For this review, take the finished solid that the model builds, in its own axes (mm). Face numbers are marked on the shaded views. Round coordinates to 2 decimals unless told otherwise and drop trailing zeros. Write each loop counter-clockwise with the first axis right and the second up, starting at its lowest first coordinate (ties: lowest second). Pieces come first, ordered by that corner, then holes. Notation, with made-up numbers: (32.5, -19.5) -> (77.5, -19.5) arc R24 cw to (77.5, 5.5) -> close; hole circle Ø5 at (23, 40). An arc over 180 degrees is marked (long way). Answer as CSV lines item,"result". Start each with the question number.
Item 1: For pin 1 Ø1.1 at (x, y) = (32, 1) entering from -Z; pin 2 Ø3 at (x, z) = (8, 8.5) entering from -Y; pin 3 Ø4 at (x, z) = (35, 3) entering from +Y, all flat-tipped, find the tip position at first contact; note any pin that passes through.
Item 2: Take a section at C-C on x = 37.5. Give the boundary of the cut face in (y, z), then the cut area to 3 significant figures.
Item 3: Take a section at A-A on x = 9. Give the boundary of the cut face in (y, z).
Item 4: Take a section at B-B on y = 0.6. Give the boundary of the cut face in (x, z), then the cut area to 3 significant figures.
Item 5: Take a section at D-D on z = 16.25. Give the boundary of the cut face in (x, y), then the cut area to 3 significant figures.
Item 6: Wall thickness on probe 1 along X at (y, z) = (1.15, 9); probe 2 along Y at (x, z) = (15, 12.75); probe 3 along X at (y, z) = (1.7, 13): over which ranges is each line inside the solid? List them lowest first. Write a range as from..to.
Item 7: Mouldability with a two-part tool opening along X and no side actions: class the marked faces 1 and 2 as +X half, -X half, draft (parallel to the pull), parting line (faces both ways), or undercut.
```python
from build123d import *

# Parameters (mm, degrees)
F0_W     = 42
F0_H     = 18
F2_DEPTH = 1.91
F1_R     = 4.6
F3_DEPTH = 3.18
F4_SIZE  = 0.25


# Not quite as in the source:
# - a feature names something its author has since deleted; it is built from what else it names


with BuildPart() as f2:
    # F0 (on Front) → F2 (new body)
    with BuildSketch(Plane.XZ):
        with Locations((21, 9)):
            Rectangle(F0_W, F0_H)
        with BuildLine():
            ThreePointArc((11.1703455946, 12.36), (9, 5), (6.8296544054, 12.36))
            ThreePointArc((6.8296544054, 12.36), (7.0893980916, 12.4791663047), (7.372240804, 12.52))
            Line((7.372240804, 12.52), (10.627759196, 12.52))
            ThreePointArc((10.627759196, 12.52), (10.9106019084, 12.4791663047), (11.1703455946, 12.36))
        make_face(mode=Mode.SUBTRACT)
        with BuildLine():
            Line((32.5, 3.2), (31.5, 3.2))
            ThreePointArc((31.5, 3.2), (27.3987806691, 4.8987806691), (25.7, 9))
            ThreePointArc((25.7, 9), (27.3987806691, 13.1012193309), (31.5, 14.8))
            Line((31.5, 14.8), (32.5, 14.8))
            ThreePointArc((32.5, 14.8), (36.6012193309, 13.1012193309), (38.3, 9))
            ThreePointArc((38.3, 9), (36.6012193309, 4.8987806691), (32.5, 3.2))
        make_face(mode=Mode.SUBTRACT)
    extrude(amount=-F2_DEPTH)

    # F1 (on face) → F3 (join)
    with BuildSketch(Plane.XZ):
        with Locations((9, 9)):
            Circle(F1_R)
        with BuildLine():
            ThreePointArc((10.627759196, 12.52), (10.9106019084, 12.4791663047), (11.1703455946, 12.36))
            ThreePointArc((11.1703455946, 12.36), (9, 5), (6.8296544054, 12.36))
            ThreePointArc((6.8296544054, 12.36), (7.0893980916, 12.4791663047), (7.372240804, 12.52))
            Line((7.372240804, 12.52), (10.627759196, 12.52))
        make_face(mode=Mode.SUBTRACT)
    extrude(amount=-F3_DEPTH)

    # F4
    f4_edges = [f2.edges().sort_by_distance(p)[0] for p in [
        (4.4, 3.18, 9),
    ]]
    chamfer(f4_edges, length=F4_SIZE)


solid = f2.part
```
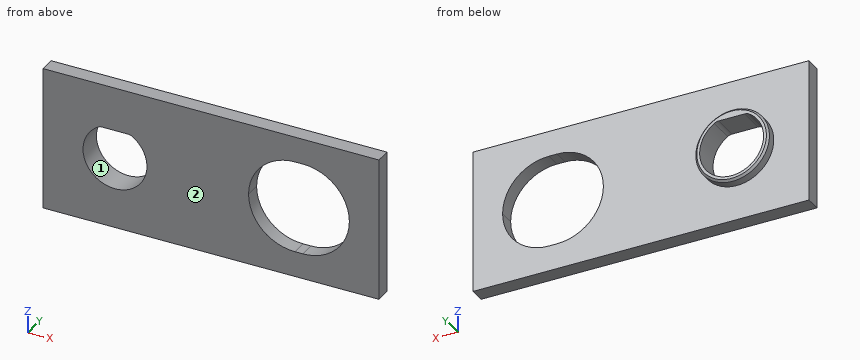
Output values:
1,pin 1,"stops at z = 0"
1,pin 2,"passes through"
1,pin 3,"stops at y = 1.91"
2,outline,"(0, 0) -> (1.91, 0) -> (1.91, 6.06) -> (0, 6.06) -> close; (0, 11.94) -> (1.91, 11.94) -> (1.91, 18) -> (0, 18) -> close"
2,area,"23.2 mm^2"
3,outline,"(0, 0) -> (1.91, 0) -> (1.91, 4.4) -> (2.93, 4.4) -> (3.18, 4.65) -> (3.18, 5) -> (0, 5) -> close; (0, 12.52) -> (3.18, 12.52) -> (3.18, 13.35) -> (2.93, 13.6) -> (1.91, 13.6) -> (1.91, 18) -> (0, 18) -> close"
4,outline,"(0, 0) -> (42, 0) -> (42, 18) -> (0, 18) -> close; hole (6.83, 12.36) arc R4 ccw (long way) to (11.17, 12.36) arc R1 ccw to (10.63, 12.52) -> (7.37, 12.52) arc R1 ccw to start; hole (31.5, 3.2) -> (32.5, 3.2) arc R5.8 ccw to (32.5, 14.8) -> (31.5, 14.8) arc R5.8 ccw to start"
4,area,"590 mm^2"
5,outline,"(0, 0) -> (42, 0) -> (42, 1.91) -> (0, 1.91) -> close"
5,area,"80.2 mm^2"
6,probe 1,"x = 0..5, 13..25.7, 38.3..42"
6,probe 2,"y = 0..1.91"
6,probe 3,"x = 0..27.3, 36.7..42"
7,face 1,"undercut"
7,face 2,"draft"
